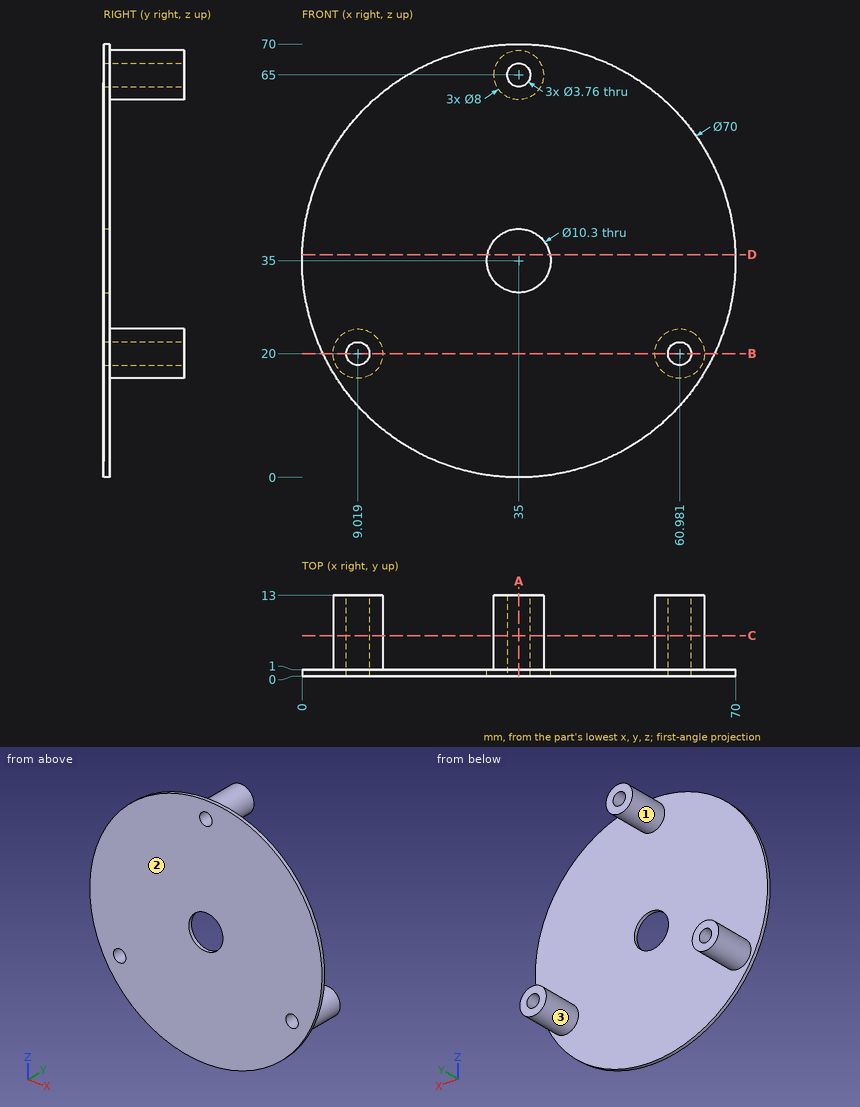
Here's the drawing with two shaded views (mm, measured from the low corner). I have some questions. Round coordinates to 2 decimals unless told otherwise and drop trailing zeros. Order: outer loops, then holes, each group sorted by start corner. A loop starts at its lowest first (then second) coordinate and runs counter-clockwise, first axis right, second up. Notation, with made-up numbers: (60.5, 3) -> (114.5, 3) arc R22 cw to (114.5, 40) -> close; hole circle Ø2 at (-8.5, -18.75). An arc over 180 degrees is marked (long way). Use a Markdown table: item, result. Add a question column.
(1) For pin 1 Ø12 at (x, z) = (35, 35) entering from +Y; pin 2 Ø4.5 at (x, z) = (35, 65) entering from +Y; pin 3 Ø4 at (y, z) = (1.5, 24.5) entering from -X; pin 4 Ø3 at (x, y) = (15.5, 10) entering from -Z, each with a flat end and sliding along its axis, tell me the tip position at first contact or that it passes through.
(2) Suppose I cut it at D-D, the plane z = 36. Please give me the cut outline in (x, y).
(3) Suppose I cut it at B-B, the plane z = 20. Please give me the cut outline in (x, y).
(4) Suppose I cut it at C-C, the plane y = 6.5. Please give me the cut outline in (x, z).
(5) If we mould it in two halves opening along X, with no side actions, what happens to the marked faces 1, 2 and 3? For each: released by +X, released by -X, zero draft, split by the parting line, or undercut.
(6) Suppose I cut it at A-A, the plane x = 35. Please give me the cut outline in (y, z).
(7) I need wall thicknesses on line 1 along Z through (x, y) = (35, 0.5); line 2 along Z through (x, y) = (9, 12.25); line 3 along X through (y, z) = (8, 20.5). Which ranges of each line are inside material? Lowest first, please.
Verdict:
| question | item | result |
|---|---|---|
| 1 | pin 1 | y = 1 |
| 1 | pin 2 | y = 13 |
| 1 | pin 3 | x = 1.06 |
| 1 | pin 4 | through |
| 2 | outline | (0.01, 0) -> (29.95, 0) -> (29.95, 1) -> (0.01, 1) -> close; (40.05, 0) -> (69.99, 0) -> (69.99, 1) -> (40.05, 1) -> close |
| 3 | outline | (3.38, 0) -> (7.14, 0) -> (7.14, 13) -> (5.02, 13) -> (5.02, 1) -> (3.38, 1) -> close; (10.9, 0) -> (59.1, 0) -> (59.1, 13) -> (56.98, 13) -> (56.98, 1) -> (13.02, 1) -> (13.02, 13) -> (10.9, 13) -> close; (62.86, 0) -> (66.62, 0) -> (66.62, 1) -> (64.98, 1) -> (64.98, 13) -> (62.86, 13) -> close |
| 4 | outline | circle Ø8 at (9.02, 20); circle Ø8 at (35, 65); circle Ø8 at (60.98, 20); hole circle Ø3.76 at (9.02, 20); hole circle Ø3.76 at (35, 65); hole circle Ø3.76 at (60.98, 20) |
| 5 | face 1 | split by the parting line |
| 5 | face 2 | zero draft |
| 5 | face 3 | undercut |
| 6 | outline | (0, 0) -> (1, 0) -> (1, 29.85) -> (0, 29.85) -> close; (0, 40.15) -> (1, 40.15) -> (1, 61) -> (13, 61) -> (13, 63.12) -> (0, 63.12) -> close; (0, 66.88) -> (13, 66.88) -> (13, 69) -> (1, 69) -> (1, 70) -> (0, 70) -> close |
| 7 | line 1 | 0 to 29.85, 40.15 to 63.12, 66.88 to 70 |
| 7 | line 2 | 16 to 18.12, 21.88 to 24 |
| 7 | line 3 | 5.05 to 7.21, 10.83 to 12.99, 57.01 to 59.17, 62.79 to 64.95 |
